Can you work these out from the model? Positions are in its coordinate system, mm. A direction names the side the tool comes from. Round coordinates to 2 decimals unless told otherwise and drop trailing zeros. Loops run counter-clockwise (first coordinate to the right, second up) from the corner with the lowest first, then second, coordinate; pieces in that order, holes last. Notation, with made-up numbers: (86, -28.5) -> (139, -28.5) arc R10 ccw to (139, -17.5) -> close; hole circle Ø6 at (-14, 51.25). An arc over 180 degrees is marked (long way). Answer as a JSON object with one key per item and string values.
```python
from build123d import *

# Parameters (mm, degrees)
BOSS_EXTRUDE1_DEPTH          = 18
SKETCH2_R                    = 1
CUT_EXTRUDE1_DEPTH           = 18
F_5_0_5_DIAMETER_HOLE1_D     = 5
F_5_0_5_DIAMETER_HOLE2_D     = 5
F_8_0_8_DIAMETER_HOLE1_D     = 8
F_8_0_8_DIAMETER_HOLE1_DEPTH = 26
F_7_0_7_DIAMETER_HOLE1_D     = 7


with BuildPart() as part:
    # Sketch1 → Boss-Extrude1 (new body)
    with BuildSketch(Plane.XY):
        Polygon((200, 234), (124, 234), (124, 303), (79, 303), (79, 365), (124, 365), (124, 434), (0, 434), (0, 0), (200, 0), align=None)
    extrude(amount=BOSS_EXTRUDE1_DEPTH)

    # Sketch2 → Cut-Extrude1 (cut)
    with BuildSketch(Plane.XY.offset(18)):
        with Locations((79, 365)):
            Circle(SKETCH2_R)
        with Locations((79, 303)):
            Circle(SKETCH2_R)
        with Locations((124, 234)):
            Circle(SKETCH2_R)
    extrude(amount=-CUT_EXTRUDE1_DEPTH, mode=Mode.SUBTRACT)

    # Ø5.0 (5) Diameter Hole1 (through all)
    with Locations(Plane.XY.offset(18)):
        with Locations((9, 397), (9, 277), (9, 157), (9, 37)):
            Hole(F_5_0_5_DIAMETER_HOLE1_D / 2)

    # Ø5.0 (5) Diameter Hole2 (through all)
    with Locations(Plane(origin=(0, 0, 0), x_dir=(-1, 0, 0), z_dir=(0, 0, -1))):
        with Locations((-191, 202), (-191, 117), (-191, 32)):
            Hole(F_5_0_5_DIAMETER_HOLE2_D / 2)

    # Ø8.0 (8) Diameter Hole1
    with Locations(Plane(origin=(124, 0, 0), x_dir=(0, 0, -1), z_dir=(1, 0, 0))):
        with Locations((-9, 398), (-9, 270)):
            Hole(F_8_0_8_DIAMETER_HOLE1_D / 2, depth=F_8_0_8_DIAMETER_HOLE1_DEPTH)

    # Ø7.0 (7) Diameter Hole1 (through all)
    with Locations(Plane.XY.offset(18)):
        with Locations((55.287909583, 361), (55.287909583, 307)):
            Hole(F_7_0_7_DIAMETER_HOLE1_D / 2)


solid = part.part
```
Q1. We'd pull the mould along Z, two halves only. Please class faces 1 (the flat face through (98, 398, 9)), 2 (the flat face through (76, 172, 0)), 3 (the flat face through (124, 399, 4.9)): pulls with the +Z half, pulls with the -Z half, needs draft (parallel to the pull), parting line crosses it, or undercut.
Determined:
{"face 1": "undercut", "face 2": "pulls with the -Z half", "face 3": "needs draft"}
Q2. I want a section at A-A, the plane x = 102. Write out the boundary of the cut face in (y, z), then the cut area to 3 significant figures.
Determined:
{"outline": "(0, 0) -> (303, 0) -> (303, 18) -> (0, 18) -> close; (365, 0) -> (434, 0) -> (434, 18) -> (365, 18) -> close; hole circle Ø8 at (270, 9); hole circle Ø8 at (398, 9)", "area": "6,600 mm²"}
Q3. I want a section at B-B, the plane z = 9. Give the number of separate pieces and of enclosed holes in the cut face, then the cut area to 3 significant figures.
Determined:
{"separate pieces": "1", "enclosed holes": "9", "area": "68,200 mm²"}
Q4. I want a section at C-C, the plane y = 251. Write out the boundary of the cut face in (x, z).
Determined:
{"outline": "(0, 0) -> (124, 0) -> (124, 18) -> (0, 18) -> close"}
Q5. On a 3-axis mill with a long thin cutter (end or side, diameter ignored), from which of +Z, -Z, +X, -X, +Y, -Y can I reach the whole of each face in a straight line? I mean faces 4 (the flat face through (102, 365, 9)), 5 (the cylindrical face through (110.818, 266.451, 10.846)), 6 (the flat face through (124, 268.5, 12.9)). Say none if no direction works.
Determined:
{"face 4": "+Z, -Z, +X", "face 5": "+X", "face 6": "+Z, -Z, +X, +Y"}
Q6. I want a section at D-D, the plane x = 129. Write out the boundary of the cut face in (y, z).
Determined:
{"outline": "(0, 0) -> (234, 0) -> (234, 18) -> (0, 18) -> close"}
Q7. I'm going to push flat-ended pins straight in: pin 1 (2.5 mm diameter, centred on x = 79, y = 365, fed in from -Z); pin 2 (4 mm diameter, centred on x = 9, y = 37, fed in from -Z); pin 3 (6 mm diameter, centred on x = 170, z = 7, fed in from +Y); pin 4 (9 mm diameter, centred on y = 270, z = 9, fed in from +X). Where does each tip first touch, or does it pass through?
Determined:
{"pin 1": "z = 0", "pin 2": "through", "pin 3": "y = 234", "pin 4": "x = 124"}
Q8. If I drill on L1, parallel to Y at x = 9, z = 5.25; L2, parallel to Y at x = 191, z = 8.5; L3, parallel to X at y = 361, z = 12.5, over which ranges is the centre line in solid material (lowest first)? Write a range as [from, to].
Determined:
{"L1": "[0, 34.5], [39.5, 154.5], [159.5, 274.5], [279.5, 394.5], [399.5, 434]", "L2": "[0, 29.5], [34.5, 114.5], [119.5, 199.5], [204.5, 234]", "L3": "[0, 51.79], [58.79, 79]"}
